```python
from build123d import *

# Parameters (mm, degrees)
ESBO_O1_R                = 5.5
RESSALTO_EXTRUS_O1_DEPTH = 40
ESBO_O2_R                = 2.65
CORTE_EXTRUS_O1_DEPTH    = 40
FILETE1_R                = 0.5
FILETE2_R                = 0.5


with BuildPart() as part:
    # Esboço1 → Ressalto-extrusão1 (new body)
    with BuildSketch(Plane(origin=(0, 0, 0), x_dir=(1, 0, 0), z_dir=(0, 1, 0))):
        with Locations(Location((0, 0, 0), (0, 0, 270))):
            Circle(ESBO_O1_R)
    extrude(amount=RESSALTO_EXTRUS_O1_DEPTH)

    # Esboço2 → Corte-extrusão1 (cut)
    with BuildSketch(Plane(origin=(0, 40, 0), x_dir=(1, 0, 0), z_dir=(0, 1, 0))):
        with Locations(Location((0, 0, 0), (0, 0, 270))):
            Circle(ESBO_O2_R)
    extrude(amount=-CORTE_EXTRUS_O1_DEPTH, mode=Mode.SUBTRACT)

    # Filete1
    filete1_edges = [part.edges().sort_by_distance(p)[0] for p in [
        (0, 0, -5.5),
        (0, 40, -5.5),
    ]]
    fillet(filete1_edges, radius=FILETE1_R)

    # Filete2
    filete2_edges = [part.edges().sort_by_distance(p)[0] for p in [
        (0, 0, -2.65),
        (0, 40, -2.65),
    ]]
    fillet(filete2_edges, radius=FILETE2_R)


solid = part.part
```
Part model, mm, in its own coordinate system. Coordinates: 2 decimals unless noted, no trailing zeros. Write each loop counter-clockwise with the first axis right and the second up, starting at its lowest first coordinate (ties: lowest second). Pieces come first, ordered by that corner, then holes.
Item 1: Slice it at A-A (z = 0). Write the cut outline in (x, y).
Item 2: Mould opens along Z. For faces 1 (the face through (-3.3, 0, -0.1)), 2 (the face through (-5.37, 19.73, -1.19)), 3 (the face through (-1.612, 20.273, -2.103)) say: released by +Z, released by -Z, zero draft, split by the parting line, or undercut.
Item 3: Pin check, flat tips, straight feed: pin 1 (2 mm diameter, centred on x = 1.5, y = 32.5, fed in from -Z); pin 2 (4 mm diameter, centred on x = -2.5, y = 30, fed in from +Z); pin 3 (2 mm diameter, centred on x = 4, y = 19, fed in from +Z). Stop position of each tip, or through.
Item 4: Slice it at B-B (x = 0). Write the cut outline in (y, z).
Item 5: Probe line 1 (X direction, y = 16, z = 0); line 2 (Y direction, x = -0.75, z = -5); line 3 (X direction, y = 16, z = -0.75). List the from-to ranges inside material, lowest first.
Item 6: Slice it at C-C (y = 20). Write the cut outline in (x, z).
Results found:
1. outline: (-5.5, 0.5) arc R0.5 ccw to (-5, 0) - (-3.15, 0) arc R0.5 ccw to (-2.65, 0.5) - (-2.65, 39.5) arc R0.5 ccw to (-3.15, 40) - (-5, 40) arc R0.5 ccw to (-5.5, 39.5) - close; (2.65, 0.5) arc R0.5 ccw to (3.15, 0) - (5, 0) arc R0.5 ccw to (5.5, 0.5) - (5.5, 39.5) arc R0.5 ccw to (5, 40) - (3.15, 40) arc R0.5 ccw to (2.65, 39.5) - close
2. face 1: zero draft
2. face 2: split by the parting line
2. face 3: undercut
3. pin 1: stops at z = -5.48
3. pin 2: stops at z = 5.48
3. pin 3: stops at z = 4.61
4. outline: (0, -5) arc R0.5 ccw to (0.5, -5.5) - (39.5, -5.5) arc R0.5 ccw to (40, -5) - (40, -3.15) arc R0.5 ccw to (39.5, -2.65) - (0.5, -2.65) arc R0.5 ccw to (0, -3.15) - close; (0, 3.15) arc R0.5 ccw to (0.5, 2.65) - (39.5, 2.65) arc R0.5 ccw to (40, 3.15) - (40, 5) arc R0.5 ccw to (39.5, 5.5) - (0.5, 5.5) arc R0.5 ccw to (0, 5) - close
5. line 1: x = -5.5 to -2.65, 2.65 to 5.5
5. line 2: y = 0 to 40
5. line 3: x = -5.45 to -2.54, 2.54 to 5.45
6. outline: circle Ø11 at (0, 0); hole circle Ø5.3 at (0, 0)
